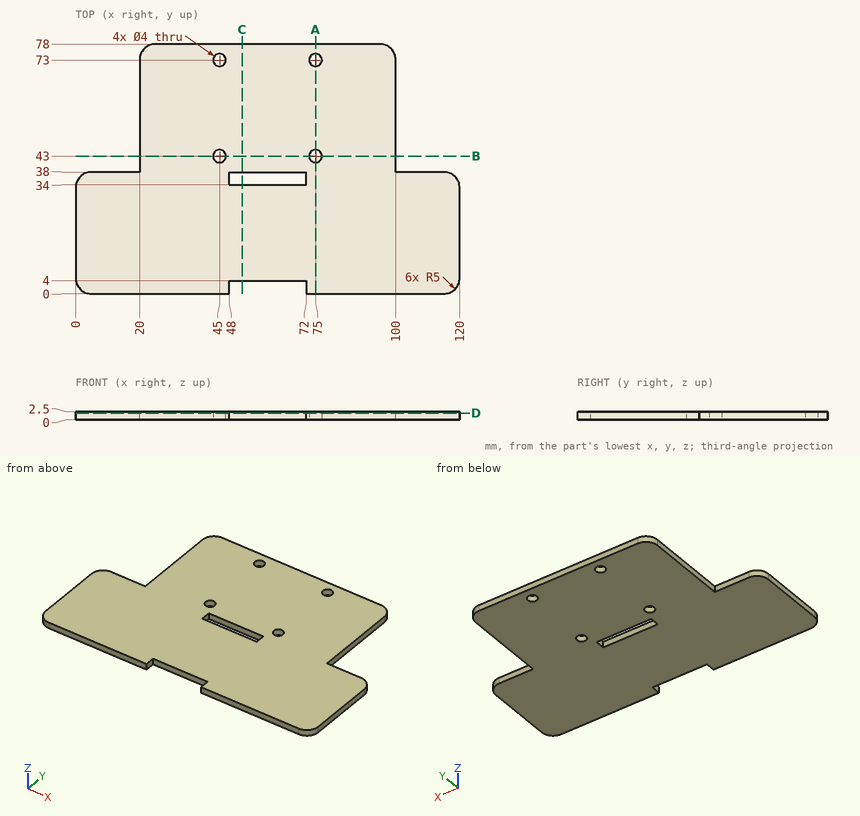
Source: three-view drawing plus pictorial views. Frame: mm from the lowest corner of the part. Coordinates: 2 decimals unless noted, no trailing zeros. Order: outer loops, then holes, each group sorted by start corner. A loop starts at its lowest first (then second) coordinate and runs counter-clockwise, first axis right, second up.
1) Section A-A (x = 75). Return loops of the section in (y, z).
Result sheet:
outline: (0, 0) - (41, 0) - (41, 2.5) - (0, 2.5) - close; (45, 0) - (71, 0) - (71, 2.5) - (45, 2.5) - close; (75, 0) - (78, 0) - (78, 2.5) - (75, 2.5) - close
2) Section D-D (z = 2.05). Return loops of the section in (x, y).
Result sheet:
outline: (0, 5) arc R5 ccw to (5, 0) - (48, 0) - (48, 4) - (72, 4) - (72, 0) - (115, 0) arc R5 ccw to (120, 5) - (120, 33) arc R5 ccw to (115, 38) - (100, 38) - (100, 73) arc R5 ccw to (95, 78) - (25, 78) arc R5 ccw to (20, 73) - (20, 38) - (5, 38) arc R5 ccw to (0, 33) - close; hole circle Ø4 at (45, 43); hole circle Ø4 at (45, 73); hole (48, 34) - (72, 34) - (72, 38) - (48, 38) - close; hole circle Ø4 at (75, 43); hole circle Ø4 at (75, 73)
3) Section B-B (y = 43). Return loops of the section in (x, z), then the cut area to 3 significant figures.
Result sheet:
outline: (20, 0) - (43, 0) - (43, 2.5) - (20, 2.5) - close; (47, 0) - (73, 0) - (73, 2.5) - (47, 2.5) - close; (77, 0) - (100, 0) - (100, 2.5) - (77, 2.5) - close
area: 180 mm2
4) Ray query, probe 1 along X at (y, z) = (73, 0.7); probe 2 along Y at (x, z) = (45, 1.95); probe 3 along X at (y, z) = (49.5, 1.25). Return the intervals inside material, ascending.
Result sheet:
probe 1: x = 20 to 43, 47 to 73, 77 to 100
probe 2: y = 0 to 41, 45 to 71, 75 to 78
probe 3: x = 20 to 100
5) Section C-C (x = 52). Return loops of the section in (y, z).
Result sheet:
outline: (4, 0) - (34, 0) - (34, 2.5) - (4, 2.5) - close; (38, 0) - (78, 0) - (78, 2.5) - (38, 2.5) - close
6) First-contact query: P1, Ø2.5, axis at x = 75, y = 73, coming from the +Z side; P2, Ø0.8, axis at x = 9.5, z = 1.5, coming from the +Y side; P3, Ø1.2, axis at y = 2.5, z = 1, coming from the +X side; P4, Ø0.8, axis at y = 36, z = 1.5, coming from the +X side. Flat tips, straight axial feed; report the tip coordinate or a pass-through.
Result sheet:
P1: passes through
P2: stops at y = 38
P3: stops at x = 119.62
P4: stops at x = 119.27
